from build123d import *

# Parameters (mm, degrees)
SKETCH_1_W                  = 150
SKETCH_1_H                  = 20
EXTRUDE_1_DEPTH             = 20
SKETCH_2_W                  = 60
SKETCH_2_H                  = 65
EXTRUDE_2_DEPTH             = 5
SKETCH_3_R                  = 1.6
CUT_EXTRUDE_1_DEPTH         = 25
SKETCH_4_W                  = 51.75
SKETCH_4_H                  = 7
CUT_EXTRUDE_2_DEPTH         = 27
SKETCH_5_R                  = 1.6
CUT_EXTRUDE_3_DEPTH         = 27
SKETCH_6_W                  = 103.5
SKETCH_6_H                  = 35
EXTRUDE_3_DEPTH             = 8
SKETCH_7_W                  = 120
SKETCH_7_H                  = 35
SKETCH_7_R                  = 3
EXTRUDE_4_DEPTH             = 3
SKETCH_8_W                  = 23.25
SKETCH_8_H                  = 20
EXTRUDE_5_DEPTH             = 3
PATTERN_LINEAR_1_COUNT      = 5
PATTERN_LINEAR_1_PITCH      = 20
PATTERN_LINEAR_1_COUNT_DIR2 = 6
PATTERN_LINEAR_1_PITCH_DIR2 = 20
EXTRUDE_6_DEPTH             = 4
SKETCH_10_W                 = 3
SKETCH_10_H                 = 23
CUT_EXTRUDE_4_DEPTH         = 29
EXTRUDE_7_DEPTH             = 40
FILLET_1_R                  = 10
FILLET_2_R                  = 3
SKETCH_16_W                 = 22
SKETCH_16_H                 = 65
SKETCH_16_R                 = 1.6
EXTRUDE_9_DEPTH             = 8.25
EXTRUDE_START               = 8.25
SKETCH_17_W                 = 22
SKETCH_17_H                 = 65
SKETCH_17_R                 = 1.6
EXTRUDE_10_DEPTH            = 8.25
FILLET_4_R                  = 5
FILLET_5_R                  = 5
FILLET_6_R                  = 1
SKETCH_18_R                 = 3
CUT_EXTRUDE_6_DEPTH         = 5
FILLET_7_R                  = 5
FILLET_8_R                  = 7
SKETCH_19_R                 = 1.6
CUT_EXTRUDE_7_DEPTH         = 45


# Some blends are built 0.0001 mm under size
with BuildPart() as part:
    # 草图1 → 凸台-拉伸1 (new body)
    with BuildSketch(Plane(origin=(0, 0, 0), x_dir=(1, 0, 0), z_dir=(0, 1, 0))):
        Rectangle(SKETCH_1_W, SKETCH_1_H)
    extrude(amount=EXTRUDE_1_DEPTH)

    # 草图2 → 凸台-拉伸2 (add)
    with BuildSketch(Plane.XY.offset(10)):
        with Locations((-30, -32.5)):
            Rectangle(SKETCH_2_W, SKETCH_2_H)
        with Locations((30, -32.5)):
            Rectangle(SKETCH_2_W, SKETCH_2_H)
    extrude(amount=-EXTRUDE_2_DEPTH)

    # 草图3 → 切除-拉伸1 (cut)
    with BuildSketch(Plane(origin=(0, 0, -10), x_dir=(-1, 0, 0), z_dir=(0, 0, -1))):
        with Locations((0, 10)):
            Circle(SKETCH_3_R)
    cut_extrude_1 = extrude(amount=-CUT_EXTRUDE_1_DEPTH, mode=Mode.SUBTRACT)

    # 草图4 → 切除-拉伸2 (cut)
    with BuildSketch(Plane(origin=(0, 20, 0), x_dir=(1, 0, 0), z_dir=(0, 1, 0))):
        with Locations((-25.875, 6.5)):
            Rectangle(SKETCH_4_W, SKETCH_4_H)
        with Locations((25.875, 6.5)):
            Rectangle(SKETCH_4_W, SKETCH_4_H)
    extrude(amount=-CUT_EXTRUDE_2_DEPTH, mode=Mode.SUBTRACT)

    # 草图5 → 切除-拉伸3 (cut)
    with BuildSketch(Plane(origin=(0, 0, 5), x_dir=(-1, 0, 0), z_dir=(0, 0, -1))):
        with Locations((43.25, -61.370748044)):
            Circle(SKETCH_5_R)
        with Locations((43.25, -39.370748224)):
            Circle(SKETCH_5_R)
        with Locations((10.750003407, -61.370748044)):
            Circle(SKETCH_5_R)
        with Locations((-17.249996593, -61.370748044)):
            Circle(SKETCH_5_R)
        with Locations((-31.749999997, -61.370748044)):
            Circle(SKETCH_5_R)
        with Locations((-31.749999997, -39.370748224)):
            Circle(SKETCH_5_R)
    extrude(amount=-CUT_EXTRUDE_3_DEPTH, mode=Mode.SUBTRACT)

    # 草图6 → 凸台-拉伸3 (add)
    with BuildSketch(Plane(origin=(0, 0, 5), x_dir=(-1, 0, 0), z_dir=(0, 0, -1))):
        with Locations((0, -17.5)):
            Rectangle(SKETCH_6_W, SKETCH_6_H)
    extrude(amount=EXTRUDE_3_DEPTH)

    # 草图7 → 凸台-拉伸4 (add)
    with BuildSketch(Plane.XY.offset(10)):
        with Locations((0, -47.5)):
            Rectangle(SKETCH_7_W, SKETCH_7_H)
        with Locations((31.749999997, -39.370748224)):
            Circle(SKETCH_7_R, mode=Mode.SUBTRACT)
        with Locations((31.749999997, -61.370748044)):
            Circle(SKETCH_7_R, mode=Mode.SUBTRACT)
        with Locations((17.249996593, -61.370748044)):
            Circle(SKETCH_7_R, mode=Mode.SUBTRACT)
        with Locations((-10.750003407, -61.370748044)):
            Circle(SKETCH_7_R, mode=Mode.SUBTRACT)
        with Locations((-43.25, -39.370748224)):
            Circle(SKETCH_7_R, mode=Mode.SUBTRACT)
        with Locations((-43.25, -61.370748044)):
            Circle(SKETCH_7_R, mode=Mode.SUBTRACT)
    extrude(amount=EXTRUDE_4_DEPTH)

    # 草图8 → 凸台-拉伸5 (add)
    with BuildSketch(Plane(origin=(0, 0, -10), x_dir=(-1, 0, 0), z_dir=(0, 0, -1))):
        with Locations((63.375, 10)):
            Rectangle(SKETCH_8_W, SKETCH_8_H)
        with Locations((-63.375, 10)):
            Rectangle(SKETCH_8_W, SKETCH_8_H)
    extrude(amount=EXTRUDE_5_DEPTH)

    # 阵列(线性)1: Cut-Extrude 1 5 × 6
    with Locations(*[Vector(1, 0, 0) * (i * PATTERN_LINEAR_1_PITCH) + Vector(-1, 0, 0) * (j * PATTERN_LINEAR_1_PITCH_DIR2) for i in range(PATTERN_LINEAR_1_COUNT) for j in range(PATTERN_LINEAR_1_COUNT_DIR2) if (i, j) != (0, 0)]):
        add(cut_extrude_1, mode=Mode.SUBTRACT)

    # 草图9 → 凸台-拉伸6 (add)
    with BuildSketch(Plane(origin=(0, 0, -13), x_dir=(-1, 0, 0), z_dir=(0, 0, -1))):
        Polygon((-75, 0), (-95, 0), (-95, 60), (-75, 60), (-75, 20), (-51.75, 20), (-51.75, 0), align=None)
        Polygon((75, 0), (95, 0), (95, 60), (75, 60), (75, 20), (51.75, 20), (51.75, 0), align=None)
    extrude(amount=EXTRUDE_6_DEPTH)

    # 草图10 → 切除-拉伸4 (cut)
    with BuildSketch(Plane(origin=(0, 20, 0), x_dir=(1, 0, 0), z_dir=(0, 1, 0))):
        with Locations((-73.5, 1.5)):
            Rectangle(SKETCH_10_W, SKETCH_10_H)
        with Locations((73.5, 1.5)):
            Rectangle(SKETCH_10_W, SKETCH_10_H)
    extrude(amount=-CUT_EXTRUDE_4_DEPTH, mode=Mode.SUBTRACT)

    # 草图11 → 凸台-拉伸7 (add)
    with BuildSketch(Plane(origin=(0, 20, 0), x_dir=(1, 0, 0), z_dir=(0, 1, 0))):
        Polygon((-69, 17), (-75, 17), (-75, 13), (-72, 13), (-72, -10), (-69, -10), align=None)
        Polygon((69, 17), (69, -10), (72, -10), (72, 13), (75, 13), (75, 17), align=None)
    extrude(amount=EXTRUDE_7_DEPTH)

    # 圆角1
    fillet_1_edges = [part.edges().sort_by_distance(p)[0] for p in [
        (-69, 20, -3.5),
        (69, 20, -3.5),
    ]]
    fillet(fillet_1_edges, radius=FILLET_1_R)

    # 圆角2
    fillet_2_edges = [part.edges().sort_by_distance(p)[0] for p in [
        (55.375, 20, -17),
        (-69, 45, -17),
        (69, 45, -17),
        (-55.375, 20, -17),
        (66.071067812, 22.928932188, -17),
        (-66.071067812, 22.928932188, -17),
        (-51.75, 20, -10),
        (51.75, 20, -10),
    ]]
    fillet(fillet_2_edges, radius=FILLET_2_R)

    # 草图16 → 凸台-拉伸9 (add)
    with BuildSketch(Plane(origin=(51.75, 0, 0), x_dir=(0, 0, -1), z_dir=(1, 0, 0))):
        with Locations((6, -32.5)):
            Rectangle(SKETCH_16_W, SKETCH_16_H)
        with Locations(Location((0.2, -39.370754998, 0), (0, 0, 270))):
            Circle(SKETCH_16_R, mode=Mode.SUBTRACT)
        with Locations(Location((0.2, -61.370748044, 0), (0, 0, 270))):
            Circle(SKETCH_16_R, mode=Mode.SUBTRACT)
    extrude(amount=EXTRUDE_9_DEPTH)

    # 草图17 → 凸台-拉伸10 (add)
    with BuildSketch(Plane.ZY.offset(51.75).offset(EXTRUDE_START)):
        with Locations((-6, -32.5)):
            Rectangle(SKETCH_17_W, SKETCH_17_H)
        with Locations(Location((-0.2, -61.370748044, 0), (0, 0, 270))):
            Circle(SKETCH_17_R, mode=Mode.SUBTRACT)
        with Locations(Location((-0.2, -39.370748224, 0), (0, 0, 270))):
            Circle(SKETCH_17_R, mode=Mode.SUBTRACT)
    extrude(amount=-EXTRUDE_10_DEPTH)

    # 圆角4
    fillet_4_edges = [part.edges().sort_by_distance(p)[0] for p in [
        (-60, 0, -3.5),
        (60, 0, -3.5),
        (95, 0, -15),
        (-95, 0, -15),
    ]]
    fillet(fillet_4_edges, radius=FILLET_4_R)

    # 圆角5
    fillet_5_edges = [part.edges().sort_by_distance(p)[0] for p in [
        (55.875, -65, -17),
        (-55.875, -65, -17),
    ]]
    fillet(fillet_5_edges, radius=FILLET_5_R)

    # 圆角6
    # the kernel refuses this fillet: 1 mm, written as the material it takes off along each edge
    with BuildSketch(Plane(origin=(62.5, -65, 13), x_dir=(0, 0, -1), z_dir=(-1, 0, 0))) as fillet_6_piece_1:
        with BuildLine():
            CenterArc((FILLET_6_R, -FILLET_6_R), FILLET_6_R, 90, 90)
            Line((0, -FILLET_6_R), (0, 0))
            Line((0, 0), (FILLET_6_R, 0))
        make_face()
    extrude(amount=125, mode=Mode.SUBTRACT)

    # 草图18 → 切除-拉伸6 (cut)
    with BuildSketch(Plane(origin=(0, 0, -3), x_dir=(-1, 0, 0), z_dir=(0, 0, -1))):
        with Locations((0, 10)):
            Circle(SKETCH_18_R)
        with Locations((20, 10)):
            Circle(SKETCH_18_R)
        with Locations((40, 10)):
            Circle(SKETCH_18_R)
        with Locations((-20, 10)):
            Circle(SKETCH_18_R)
        with Locations((-40, 10)):
            Circle(SKETCH_18_R)
    extrude(amount=-CUT_EXTRUDE_6_DEPTH, mode=Mode.SUBTRACT)

    # 圆角7
    fillet_7_edges = [part.edges().sort_by_distance(p)[0] for p in [
        (0, -35, -3),
    ]]
    fillet(fillet_7_edges, radius=FILLET_7_R)

    # 圆角8
    fillet_8_edges = [part.edges().sort_by_distance(p)[0] for p in [
        (-72, 0, -1.5),
        (72, 0, -1.5),
    ]]
    fillet(fillet_8_edges, radius=FILLET_8_R - 0.0001)  # a hair under: the kernel refuses the full size

    # 草图19 → 切除-拉伸7 (cut)
    with BuildSketch(Plane.XY.offset(13)):
        with Locations((85, 39.999999445)):
            Circle(SKETCH_19_R)
        with Locations((85, 19.999999445)):
            Circle(SKETCH_19_R)
        with Locations((-85, 19.999999445)):
            Circle(SKETCH_19_R)
        with Locations((-85, 39.999999445)):
            Circle(SKETCH_19_R)
    extrude(amount=-CUT_EXTRUDE_7_DEPTH, mode=Mode.SUBTRACT)


solid = part.part
Input: part model. Units: mm. Frame: model coordinates. A direction names the side the tool comes from. Coordinates: 2 decimals unless noted, no trailing zeros. Order: outer loops, then holes, each group sorted by start corner. A loop starts at its lowest first (then second) coordinate and runs counter-clockwise, first axis right, second up. Notation, with made-up numbers: M 39,60.25 L 94,60.25 A22 cw 94,74.25 Z; hole C 73.5,25 d9. An arc over 180 degrees is marked long. Answer in a Markdown table with one row per item.
(1) Draft query along X for faces 1 (the cylindrical face through (62, -1, -3)), 2 (the cylindrical face through (-37, 10, -1)), 3 (the flat face through (-0.8, -65, 5.2)), 4 (the flat face through (-60, -35, -2)). Return one class per face: pulls with the +X half, pulls with the -X half, needs draft (parallel to the pull), parting line crosses it, or undercut.
Numbers:
| item | result |
|---|---|
| face 1 | pulls with the +X half |
| face 2 | undercut |
| face 3 | needs draft |
| face 4 | pulls with the -X half |
(2) Access query for faces 5 (the cylindrical face through (65.99, 22.85, -1.83)), 6 (the flat face through (33, -38, 10)), 7 (the flat face through (51.75, -23, -8)), 8 (the cylindrical face through (-17, 10, -1)). Directions: +Z, -Z, +X, -X, +Y, -Y. A direction counts if a zero-diameter tool reaches every point of the face in a straight line with its end or side. Return the directions, or none.
Numbers:
| item | result |
|---|---|
| face 5 | +Z, -Z, +Y |
| face 6 | +Z |
| face 7 | -Z, -Y |
| face 8 | -Z |
(3) Section query A-A, the plane z = -5.5. Give the number of separate pieces and of enclosed holes in the cut face, plus the area to 3 significant figures.
Numbers:
| item | result |
|---|---|
| separate pieces | 2 |
| enclosed holes | 2 |
| area | 2,140 mm^2 |
(4) Section query C-C, the plane y = -24. Output: boundary loops of the cut face in (x, z).
Numbers:
| item | result |
|---|---|
| outline | M -60,-17 L -51.75,-17 L -51.75,-3 L 51.75,-3 L 51.75,-17 L 60,-17 L 60,10 L -60,10 Z |
(5) Contact query for flat-ended pins moving along their axis: pin 1 Ø3.5 at (x, z) = (-5.5, 11) entering from +Y; pin 2 Ø3 at (x, z) = (0.5, 4.5) entering from -Y; pin 3 Ø12 at (x, y) = (3, 0.5) entering from +Z; pin 4 Ø5.5 at (x, y) = (-20, 10) entering from -Z. Output: stop coordinate, or through.
Numbers:
| item | result |
|---|---|
| pin 1 | stops at y = 20 |
| pin 2 | stops at y = -65 |
| pin 3 | stops at z = 10 |
| pin 4 | stops at z = 2 |
(6) Section query B-B, the plane y = 46.5. Output: boundary loops of the cut face in (x, z).
Numbers:
| item | result |
|---|---|
| outline | M -95,-17 L -72,-17 A3 ccw -69,-14 L -69,10 L -72,10 L -72,-13 L -95,-13 Z; M 69,-14 A3 ccw 72,-17 L 95,-17 L 95,-13 L 72,-13 L 72,10 L 69,10 Z |
(7) Material intervals for line 1 (Y direction, x = 54, z = 0); line 2 (X direction, y = -39, z = -11.5); line 3 (Y direction, x = 0, z = 7.75), sorted ascending. Write a range as [from, to].
Numbers:
| item | result |
|---|---|
| line 1 | y = [-65, -62.96], [-59.78, -40.96], [-37.78, 20] |
| line 2 | x = [-60, -51.75], [51.75, 60] |
| line 3 | y = [-65, 8.4], [11.6, 20] |
